Solid Edge part; units mm, degrees
sketch "Sketch1" plane through (0, 0, 0) normal (0, 0, 1) x (1, 0, 0)
  circle A0 centre (0, 0) radius 10.5
  circle A1 centre (0, 0) radius 5.5
extrude "Protrusion1" add sketch "Sketch1" along normal blind 3
sketch "Sketch2" plane through (0, 0, 0) normal (0, 0, -1) x (1, 0, 0)
  circle A0 centre (0, 0) radius 6.5
extrude "ExtrudedCutout_1" cut sketch "Sketch2" against normal blind 2.7
hole "Hole_1" at (0, 9, 0) direction (0, 0, 1) diameter 2.2 end up to next
pattern_circular "Pattern1" count 4 over 360 about axis through (0, 0, 0) along (0, 0, 1) of "Hole_1"
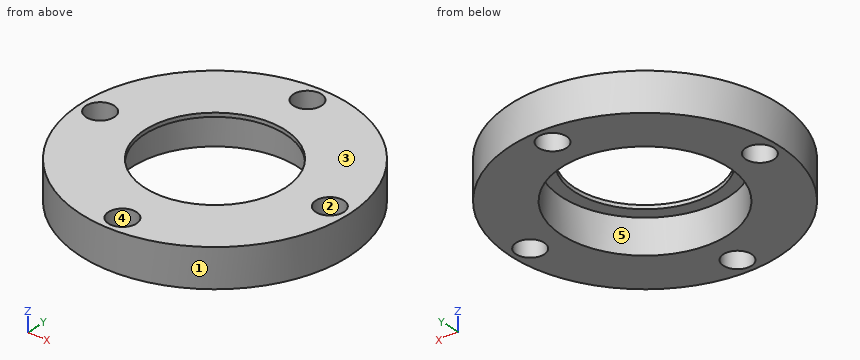
Can you work these out from the model? Positions are in its coordinate system, mm. Face numbers are marked on the shaded views. A direction names the side the tool comes from. Coordinates: 2 decimals unless noted, no trailing zeros. Loops run counter-clockwise (first coordinate to the right, second up) from the corner with the lowest first, then second, coordinate; pieces in that order, holes last.
1) Imagine slicing it at A-A on x = 0. List the corners of the cut face in (y, z) for me.
2) Imagine slicing it at C-C on y = 3.5. List the corners of the cut face in (x, z) for me.
3) Which directions (+Z, -Z, +X, -X, +Y, -Y) give clear straight access to the entire face, cutting with the end or side of a thin tool? Please do the marked faces 4 and 5.
4) Imagine slicing it at B-B on z = 1.15. List the corners of the cut face in (x, y) for me, plus the area to 3 significant figures.
5) I need wall thicknesses on probe 1 along Y at (x, z) = (0, 2.3); probe 2 along X at (y, z) = (0.5, 2.45). Which ranges of each line are inside material? Lowest first, please.
6) Thinking about a two-plate mould opening in X: for the marked faces 1, 2 and 3, which applies, pulls with the +X half, pulls with the -X half, needs draft (parallel to the pull), parting line crosses it, or undercut?
7) For pin 1 (6.5 mm diameter, centred on x = 0, y = 0.5, fed in from -Z); pin 2 (1.5 mm diameter, centred on y = -8, z = 0.5, fed in from -X); pin 3 (12.5 mm diameter, centred on x = 0, y = 0, fed in from -Z); pin 4 (1 mm diameter, centred on y = -5, z = 1, fed in from +X), each with a flat end and sliding along its axis, tell me the tip position at first contact or that it passes through.
Completed:
1. outline: (-10.5, 0) - (-10.1, 0) - (-10.1, 3) - (-10.5, 3) - close; (-7.9, 0) - (-6.5, 0) - (-6.5, 2.7) - (-5.5, 2.7) - (-5.5, 3) - (-7.9, 3) - close; (5.5, 2.7) - (6.5, 2.7) - (6.5, 0) - (7.9, 0) - (7.9, 3) - (5.5, 3) - close; (10.1, 0) - (10.5, 0) - (10.5, 3) - (10.1, 3) - close
2. outline: (-9.9, 0) - (-5.48, 0) - (-5.48, 2.7) - (-4.24, 2.7) - (-4.24, 3) - (-9.9, 3) - close; (4.24, 2.7) - (5.48, 2.7) - (5.48, 0) - (9.9, 0) - (9.9, 3) - (4.24, 3) - close
3. face 4: +Z, -Z
3. face 5: -Z
4. outline: circle Ø21 at (0, 0); hole circle Ø2.2 at (-9, 0); hole circle Ø13 at (0, 0); hole circle Ø2.2 at (0, -9); hole circle Ø2.2 at (0, 9); hole circle Ø2.2 at (9, 0)
4. area: 198 mm2
5. probe 1: y = -10.5 to -10.1, -7.9 to -6.5, 6.5 to 7.9, 10.1 to 10.5
5. probe 2: x = -10.49 to -9.98, -8.02 to -6.48, 6.48 to 8.02, 9.98 to 10.49
6. face 1: parting line crosses it
6. face 2: undercut
6. face 3: needs draft
7. pin 1: passes through
7. pin 2: stops at x = -7.6
7. pin 3: stops at z = 2.7
7. pin 4: stops at x = 9.49
